```python
from build123d import *

# Parameters (mm, degrees)
SKETCH1_R           = 6.5
BOSS_EXTRUDE1_DEPTH = 4
SKETCH4_R           = 2.6
CUT_EXTRUDE1_DEPTH  = 10
SKETCH5_W           = 200
SKETCH5_H           = 4
BOSS_EXTRUDE2_DEPTH = 100
FILLET1_R           = 4
RIB5_START          = -2
RIB5_DEPTH          = 4
SKETCH8_R           = 5
CUT_EXTRUDE4_DEPTH  = 100
SKETCH11_R          = 2.6
CUT_EXTRUDE7_DEPTH  = 40
SKETCH9_R           = 5
CUT_EXTRUDE8_DEPTH  = 10
SKETCH12_R          = 1.978720795
SKETCH12_R_2        = 1.75
CUT_EXTRUDE9_DEPTH  = 10


# Read off the part's stored shape, not the designer's step: Rib5
with BuildPart() as part:
    # Sketch1 → Boss-Extrude1 (new body)
    with BuildSketch(Plane.XY):
        with BuildLine():
            Line((100, 0), (37.87398813, 182.867051841))
            ThreePointArc((37.87398813, 182.867051841), (0, 210), (-37.87398813, 182.867051841))
            Line((-37.87398813, 182.867051841), (-100, 0))
            Line((-100, 0), (-100, -4))
            Line((-100, -4), (100, -4))
            Line((100, -4), (100, 0))
        make_face()
        with Locations((0, 170)):
            Circle(SKETCH1_R, mode=Mode.SUBTRACT)
    extrude(amount=BOSS_EXTRUDE1_DEPTH)

    # Sketch4 → Cut-Extrude1 (cut)
    with BuildSketch(Plane(origin=(0, 0, 0), x_dir=(-1, 0, 0), z_dir=(0, 0, -1))):
        with Locations((0, 188.25)):
            Circle(SKETCH4_R)
        with Locations((0, 151.75)):
            Circle(SKETCH4_R)
    extrude(amount=-CUT_EXTRUDE1_DEPTH, mode=Mode.SUBTRACT)

    # Sketch5 → Boss-Extrude2 (add)
    with BuildSketch(Plane(origin=(0, 0, 0), x_dir=(-1, 0, 0), z_dir=(0, 0, -1))):
        with Locations((0, -2)):
            Rectangle(SKETCH5_W, SKETCH5_H)
    extrude(amount=-BOSS_EXTRUDE2_DEPTH)

    # Fillet1
    fillet1_edges = [part.edges().sort_by_distance(p)[0] for p in [
        (0, -4, 0),
        (0, 0, 4),
    ]]
    fillet(fillet1_edges, radius=FILLET1_R)

    # Rib5 outline → Rib5 (add)
    with BuildSketch(Plane.YZ.offset(RIB5_START)):
        with BuildLine():
            Line((4, 4), (100, 4))
            Line((100, 4), (0, 84))
            Line((0, 84), (0, 8))
            ThreePointArc((0, 8), (1.171572875, 5.171572875), (4, 4))
        make_face()
    extrude(amount=RIB5_DEPTH)

    # Sketch8 → Cut-Extrude4 (cut)
    with BuildSketch(Plane(origin=(0, 0, 0), x_dir=(1, 0, 0), z_dir=(0, 1, 0))):
        with Locations(Location((-75, -80, 0), (0, 0, 270))):
            Circle(SKETCH8_R)
        with Locations(Location((-75, -20, 0), (0, 0, 270))):
            Circle(SKETCH8_R)
        with Locations(Location((75, -80, 0), (0, 0, 270))):
            Circle(SKETCH8_R)
        with Locations(Location((75, -20, 0), (0, 0, 270))):
            Circle(SKETCH8_R)
    extrude(amount=-CUT_EXTRUDE4_DEPTH, mode=Mode.SUBTRACT)

    # Sketch11 → Cut-Extrude7 (cut)
    with BuildSketch(Plane(origin=(0, 0, 0), x_dir=(-1, 0, 0), z_dir=(0, 0, -1))):
        with Locations((-18.25, 65)):
            Circle(SKETCH11_R)
        with Locations((18.25, 65)):
            Circle(SKETCH11_R)
    extrude(amount=-CUT_EXTRUDE7_DEPTH, mode=Mode.SUBTRACT)

    # Sketch9 → Cut-Extrude8 (cut)
    with BuildSketch(Plane.XY.offset(4)):
        with Locations((-35, 21)):
            Circle(SKETCH9_R)
        with Locations((35, 21)):
            Circle(SKETCH9_R)
    extrude(amount=-CUT_EXTRUDE8_DEPTH, mode=Mode.SUBTRACT)

    # Sketch12 → Cut-Extrude9 (cut)
    with BuildSketch(Plane.XY.offset(4)):
        with Locations((-15.5, 185.5)):
            Circle(SKETCH12_R)
        with Locations((15.5, 185.5)):
            Circle(SKETCH12_R)
        with Locations((15.5, 154.5)):
            Circle(SKETCH12_R)
        with Locations((-15.5, 154.5)):
            Circle(SKETCH12_R_2)
    extrude(amount=-CUT_EXTRUDE9_DEPTH, mode=Mode.SUBTRACT)


solid = part.part
```
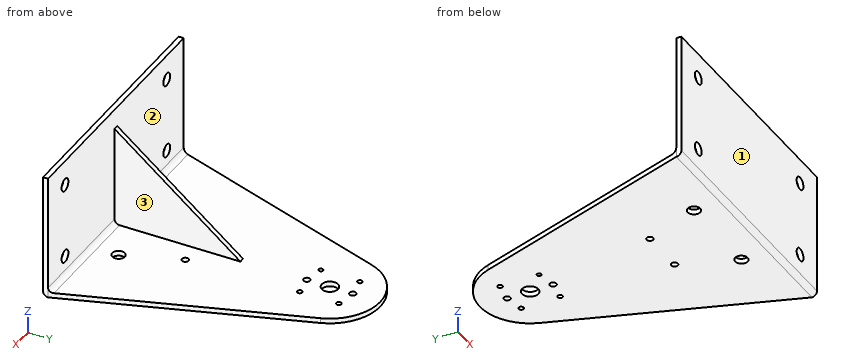
Here's how the part is built. I have some questions about the finished solid (model axes, mm). Face numbers are marked on the shaded views. A direction names the side the tool comes from. Give positions to 0.01 mm unless a question says otherwise; leave off trailing zeros. Loops run counter-clockwise (first coordinate to the right, second up) from the corner with the lowest first, then second, coordinate; pieces in that order, holes last. Notation, with made-up numbers: M 62,51 L 69,51 A4 ccw 69,55 Z; hole C -17,80 d7. An arc over 180 degrees is marked long. Use one line per item in the form item = value. Start each with the question number.
Q1. Will these pins go through, and if not, where does the flat tip stop? pin 1 Ø4.5 at (x, y) = (0, 151.75) entering from +Z; pin 2 Ø24 at (y, z) = (43.5, 60) entering from -X; pin 3 Ø10 at (x, y) = (-34.5, 101.5) entering from +Z; pin 4 Ø1.5 at (x, z) = (58, 78) entering from +Y.
Q2. Which directions (+Z, -Z, +X, -X, +Y, -Y) give clear straight access to the entire face, cutting with the end or side of a thin tool? Please do the marked faces 1, 2 and 3.
Q3. If we section it at A-A (z = 80): Write out the boundary of the cut face in (x, y), then the cut area to 3 significant figures.
Q4. If we section it at B-B (x = 35): Write out the boundary of the cut face in (y, z).
Q5. If we section it at C-C (x = -75): Write out the boundary of the cut face in (y, z), then the cut area to 3 significant figures.
Q6. If we section it at D-D (z = 35): Write out the boundary of the cut face in (x, y), then the cut area to 4 significant figures.
Q7. I need wall thicknesses on line 1 along X through (y, z) = (-1.95, 80); line 2 along Y through (x, z) = (0, 1.7); line 3 along Y through (x, z) = (0, 1.25). Which ranges of each line are inside material? Lowest first, please.
Taken from the geometry:
q1.pin_1 = through
q1.pin_2 = -2
q1.pin_3 = 4
q1.pin_4 = 0
q2.face_1 = +Z, -Z, +X, -X, -Y
q2.face_2 = +Z, +Y
q2.face_3 = +Z, +X, +Y
q3.outline = M -100,-4 L -80,-4 L -80,0 L -100,0 Z; M -70,-4 L 70,-4 L 70,0 L 2,0 L 2,5 L -2,5 L -2,0 L -70,0 Z; M 80,-4 L 100,-4 L 100,0 L 80,0 Z
q3.area = 740 mm^2
q4.outline = M -4,4 A4 ccw 0,0 L 16,0 L 16,4 L 4,4 A4 cw 0,8 L 0,100 L -4,100 Z; M 26,0 L 189.36,0 L 189.36,4 L 26,4 Z
q5.outline = M -4,4 A4 ccw 0,0 L 73.59,0 L 73.59,4 L 4,4 A4 cw 0,8 L 0,15 L -4,15 Z; M -4,25 L 0,25 L 0,75 L -4,75 Z; M -4,85 L 0,85 L 0,100 L -4,100 Z
q5.area = 614 mm^2
q6.outline = M -100,-4 L 100,-4 L 100,0 L 2,0 L 2,61.25 L -2,61.25 L -2,0 L -100,0 Z
q6.area = 1,045 mm^2
q7.line_1 = -100 to -80, -70 to 70, 80 to 100
q7.line_2 = -3.27 to 149.15, 154.35 to 163.5, 176.5 to 185.65, 190.85 to 210
q7.line_3 = -2.9 to 149.15, 154.35 to 163.5, 176.5 to 185.65, 190.85 to 210
